Read the model definition and answer for the solid it produces. Units are mm, in the model's axes. Coordinates: 2 decimals unless noted, no trailing zeros. Loops run counter-clockwise (first coordinate to the right, second up) from the corner with the lowest first, then second, coordinate; pieces in that order, holes last. Notation, with made-up numbers: M 58.5,18.5 L 101.5,18.5 A34 cw 101.5,50.5 Z; hole C 51,26 d9. An arc over 180 degrees is marked long. Use one line per item in the form item = value. Start each with the question number.
1. The part is cut by section B-B (y = 3.4). Give the number of separate pieces and of enclosed holes in the cut face, plus the area to 3 significant figures.
2. Find the intervals of material crossed by probe 1 along X at (y, z) = (3.35, 0) (3 decimals); probe 2 along X at (y, z) = (4.5, 1.5) (3 decimals); probe 3 along Z at (x, y) = (-26, 4.35), in increasing order. Write a range as [from, to].
3. For a pull along Z with two mould halves and no side action, classify faces 1 (the flat face through (-1, 2, -19.05)), 2 (the flat face through (53.975, 2, 0)), 3 (the cylindrical face through (37.26, 2.35, 6.96)) as released by +Z, released by -Z, zero draft, split by the parting line, or undercut.
4. The part is cut by section A-A (z = 0). Give the vertices of the cut face in (x, y) (1 decimal).
from build123d import *

# Parameters (mm, degrees)
SKETCH2_W           = 107.95
SKETCH2_H           = 38.1
SKETCH2_R           = 4.7625
BOSS_EXTRUDE1_DEPTH = 4.7625
SKETCH3_R           = 2.54
SKETCH3_R_2         = 6.35
CUT_EXTRUDE1_DEPTH  = 58.435916736


with BuildPart() as part:
    # Sketch2 → Boss-Extrude1 (new body)
    with BuildSketch(Plane(origin=(0, 0, 0), x_dir=(1, 0, 0), z_dir=(0, 1, 0))):
        Rectangle(SKETCH2_W, SKETCH2_H)
        with Locations(Location((41.275, 9.525, 0), (0, 0, 90))):
            Circle(SKETCH2_R, mode=Mode.SUBTRACT)
        with Locations(Location((41.275, -9.525, 0), (0, 0, 90))):
            Circle(SKETCH2_R, mode=Mode.SUBTRACT)
    extrude(amount=BOSS_EXTRUDE1_DEPTH)

    # Sketch3 → Cut-Extrude1 (cut, through all)
    with BuildSketch(Plane(origin=(0, 4.7625, 0), x_dir=(1, 0, 0), z_dir=(0, 1, 0))):
        with Locations(Location((-39.497, 0, 0), (0, 0, 270))):
            Circle(SKETCH3_R)
        with Locations(Location((-2.413, 0, 0), (0, 0, 270))):
            Circle(SKETCH3_R)
        with Locations(Location((-20.955, 0, 0), (0, 0, 270))):
            Circle(SKETCH3_R_2)
    extrude(amount=-CUT_EXTRUDE1_DEPTH, mode=Mode.SUBTRACT)


solid = part.part
Computed values:
q1.separate_pieces = 1
q1.enclosed_holes = 5
q1.area = 3,800 mm²
q2.probe_1 = [-53.975, -42.037], [-36.957, -27.305], [-14.605, -4.953], [0.127, 53.975]
q2.probe_2 = [-53.975, -41.547], [-37.447, -27.125], [-14.785, -4.463], [-0.363, 53.975]
q2.probe_3 = [-19.05, -3.86], [3.86, 19.05]
q3.face_1 = released by -Z
q3.face_2 = zero draft
q3.face_3 = undercut
q4.outline = M -54,0 L -42,0 L -42,4.8 L -54,4.8 Z; M -37,0 L -27.3,0 L -27.3,4.8 L -37,4.8 Z; M -14.6,0 L -5,0 L -5,4.8 L -14.6,4.8 Z; M 0.1,0 L 54,0 L 54,4.8 L 0.1,4.8 Z
